Input: part model. Units: mm. Frame: model coordinates. Round coordinates to 2 decimals unless told otherwise and drop trailing zeros. Order: outer loops, then holes, each group sorted by start corner. A loop starts at its lowest first (then second) coordinate and runs counter-clockwise, first axis right, second up. Notation, with made-up numbers: (-1, 21) -> (17, 21) arc R31 cw to (17, 59) -> close; hole circle Ø2 at (36, 31.5). An arc over 180 degrees is marked (long way). Answer as CSV lines item,"result". Start each with the question number.
1) Section query B-B, the plane x = -19.5. Output: boundary loops of the cut face in (y, z).
2) Line query: L1, parallel to Y at x = -20, z = 0.3; L2, parallel to X at y = -4, z = 0.95; L3, parallel to X at y = -10.5, z = 0.35. Output: solid intervals per line, ascending.
3) Section query D-D, the plane y = 0. Output: boundary loops of the cut face in (x, z), and give its area (3 significant figures).
4) Section query C-C, the plane y = -20. Output: boundary loops of the cut face in (x, z), and give its area (3 significant figures).
5) Section query A-A, the plane z = 0.55. Output: boundary loops of the cut face in (x, y).
6) First-contact query: P1, Ø4, axis at x = -20, y = -20, coming from the -Z side. Flat tip, straight axial feed; report the tip coordinate or a pass-through.
```python
from build123d import *

# Parameters (mm, degrees)
SKETCH1_R           = 2.65
BOSS_EXTRUDE1_DEPTH = 1


with BuildPart() as part:
    # Sketch1 → Boss-Extrude1 (new body)
    with BuildSketch(Plane.XY):
        with BuildLine():
            Line((-10.16, 33.49290074), (10.16, 33.49290074))
            ThreePointArc((10.16, 33.49290074), (27.504846413, 21.644477906), (34.942810419, 2))
            ThreePointArc((34.942810419, 2), (32.999182505, 0), (34.942810419, -2))
            ThreePointArc((34.942810419, -2), (27.504846413, -21.644477906), (10.16, -33.49290074))
            Line((10.16, -33.49290074), (-10.16, -33.49290074))
            ThreePointArc((-10.16, -33.49290074), (-27.504846413, -21.644477906), (-34.942810419, -2))
            ThreePointArc((-34.942810419, -2), (-32.999182505, 0), (-34.942810419, 2))
            ThreePointArc((-34.942810419, 2), (-27.504846413, 21.644477906), (-10.16, 33.49290074))
        make_face()
        with Locations((-20, 20)):
            Circle(SKETCH1_R, mode=Mode.SUBTRACT)
        with Locations((-20, -20)):
            Circle(SKETCH1_R, mode=Mode.SUBTRACT)
        with Locations((20, -20)):
            Circle(SKETCH1_R, mode=Mode.SUBTRACT)
        with Locations((20, 20)):
            Circle(SKETCH1_R, mode=Mode.SUBTRACT)
    extrude(amount=BOSS_EXTRUDE1_DEPTH)


solid = part.part
```
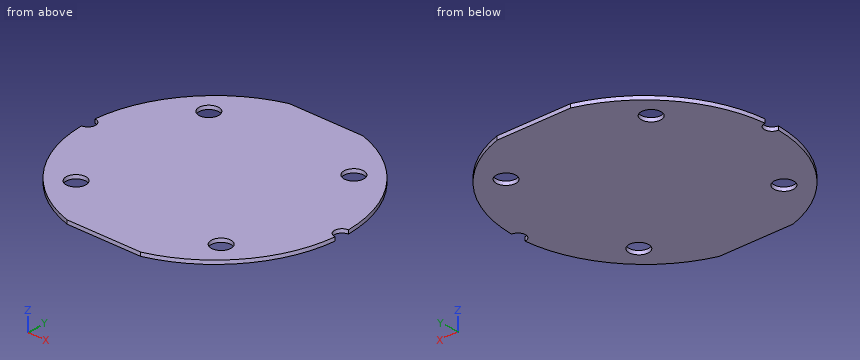
Findings:
1,outline,"(-29.06, 0) -> (-22.6, 0) -> (-22.6, 1) -> (-29.06, 1) -> close; (-17.4, 0) -> (17.4, 0) -> (17.4, 1) -> (-17.4, 1) -> close; (22.6, 0) -> (29.06, 0) -> (29.06, 1) -> (22.6, 1) -> close"
2,L1,"y = -28.72 to -22.65, -17.35 to 17.35, 22.65 to 28.72"
2,L2,"x = -34.77 to 34.77"
2,L3,"x = -33.39 to 33.39"
3,outline,"(-33, 0) -> (33, 0) -> (33, 1) -> (-33, 1) -> close"
3,area,"66.0 mm^2"
4,outline,"(-28.72, 0) -> (-22.65, 0) -> (-22.65, 1) -> (-28.72, 1) -> close; (-17.35, 0) -> (17.35, 0) -> (17.35, 1) -> (-17.35, 1) -> close; (22.65, 0) -> (28.72, 0) -> (28.72, 1) -> (22.65, 1) -> close"
4,area,"46.8 mm^2"
5,outline,"(-34.94, -2) arc R35 ccw to (-10.16, -33.49) -> (10.16, -33.49) arc R35 ccw to (34.94, -2) arc R2 cw to (34.94, 2) arc R35 ccw to (10.16, 33.49) -> (-10.16, 33.49) arc R35 ccw to (-34.94, 2) arc R2 cw to start; hole circle Ø5.3 at (-20, -20); hole circle Ø5.3 at (-20, 20); hole circle Ø5.3 at (20, -20); hole circle Ø5.3 at (20, 20)"
6,P1,"passes through"
